```python
from build123d import *

# Parameters (mm, degrees)
SKETCH_1_R      = 1.5
SKETCH_1_R_2    = 1.45
EXTRUDE_1_DEPTH = 4


with BuildPart() as part:
    # 草圖1 → 填料-伸長1 (new body)
    with BuildSketch(Plane(origin=(0, 4, 0), x_dir=(1, 0, 0), z_dir=(0, 1, 0))):
        Polygon((-75, 160.5), (-90, 190.5), (-110, 190.5), (-110, -190.5), (110, -190.5), (110, 190.5), (90, 190.5), (75, 160.5), align=None)
        with Locations((79.5, -32.625)):
            Circle(SKETCH_1_R, mode=Mode.SUBTRACT)
        with Locations((79.5, -140.625)):
            Circle(SKETCH_1_R, mode=Mode.SUBTRACT)
        with Locations((-75, 132.5)):
            Circle(SKETCH_1_R_2, mode=Mode.SUBTRACT)
        with Locations((1.6, 132.5)):
            Circle(SKETCH_1_R_2, mode=Mode.SUBTRACT)
        with Locations((-75, 70.78)):
            Circle(SKETCH_1_R_2, mode=Mode.SUBTRACT)
        with Locations((1.6, 70.78)):
            Circle(SKETCH_1_R_2, mode=Mode.SUBTRACT)
        with Locations((1.6, 55.5)):
            Circle(SKETCH_1_R_2, mode=Mode.SUBTRACT)
        with Locations((-75, 55.5)):
            Circle(SKETCH_1_R_2, mode=Mode.SUBTRACT)
        with Locations((-75, -6.22)):
            Circle(SKETCH_1_R_2, mode=Mode.SUBTRACT)
        with Locations((1.6, -6.22)):
            Circle(SKETCH_1_R_2, mode=Mode.SUBTRACT)
        with Locations((-75, -21.5)):
            Circle(SKETCH_1_R_2, mode=Mode.SUBTRACT)
        with Locations((1.6, -21.5)):
            Circle(SKETCH_1_R_2, mode=Mode.SUBTRACT)
        with Locations((-75, -83.22)):
            Circle(SKETCH_1_R_2, mode=Mode.SUBTRACT)
        with Locations((1.6, -83.22)):
            Circle(SKETCH_1_R_2, mode=Mode.SUBTRACT)
        with Locations((1.6, -98.5)):
            Circle(SKETCH_1_R_2, mode=Mode.SUBTRACT)
        with Locations((-75, -98.5)):
            Circle(SKETCH_1_R_2, mode=Mode.SUBTRACT)
        with Locations((-75, -160.22)):
            Circle(SKETCH_1_R_2, mode=Mode.SUBTRACT)
        with Locations((1.6, -160.22)):
            Circle(SKETCH_1_R_2, mode=Mode.SUBTRACT)
        with Locations((-28.86, -181.5)):
            Circle(SKETCH_1_R_2, mode=Mode.SUBTRACT)
        with Locations((78.5, -181.5)):
            Circle(SKETCH_1_R_2, mode=Mode.SUBTRACT)
        with BuildLine():
            Line((-104, 1.5), (-102, 1.5))
            ThreePointArc((-102, 1.5), (-100.5, 0), (-102, -1.5))
            Line((-102, -1.5), (-104, -1.5))
            ThreePointArc((-104, -1.5), (-105.5, 0), (-104, 1.5))
        make_face(mode=Mode.SUBTRACT)
        with BuildLine():
            Line((102, -116), (104, -116))
            ThreePointArc((104, -116), (105.5, -117.5), (104, -119))
            Line((104, -119), (102, -119))
            ThreePointArc((102, -119), (100.5, -117.5), (102, -116))
        make_face(mode=Mode.SUBTRACT)
        with BuildLine():
            Line((102, 1.5), (104, 1.5))
            ThreePointArc((104, 1.5), (105.5, 0), (104, -1.5))
            Line((104, -1.5), (102, -1.5))
            ThreePointArc((102, -1.5), (100.5, 0), (102, 1.5))
        make_face(mode=Mode.SUBTRACT)
        with BuildLine():
            Line((102, 119), (104, 119))
            ThreePointArc((104, 119), (105.5, 117.5), (104, 116))
            Line((104, 116), (102, 116))
            ThreePointArc((102, 116), (100.5, 117.5), (102, 119))
        make_face(mode=Mode.SUBTRACT)
        with BuildLine():
            Line((-104, -116), (-102, -116))
            ThreePointArc((-102, -116), (-100.5, -117.5), (-102, -119))
            Line((-102, -119), (-104, -119))
            ThreePointArc((-104, -119), (-105.5, -117.5), (-104, -116))
        make_face(mode=Mode.SUBTRACT)
        with BuildLine():
            Line((-104, 119), (-102, 119))
            ThreePointArc((-102, 119), (-100.5, 117.5), (-102, 116))
            Line((-102, 116), (-104, 116))
            ThreePointArc((-104, 116), (-105.5, 117.5), (-104, 119))
        make_face(mode=Mode.SUBTRACT)
        Polygon((15.6, 132.5), (57.6, 132.5), (62.6, 127.5), (62.6, 75.78), (57.6, 70.78), (15.6, 70.78), align=None, mode=Mode.SUBTRACT)
        Polygon((57.6, 55.5), (62.6, 50.5), (62.6, -1.22), (57.6, -6.22), (15.6, -6.22), (15.6, 55.5), align=None, mode=Mode.SUBTRACT)
        Polygon((57.6, -21.5), (62.6, -26.5), (62.6, -78.22), (57.6, -83.22), (15.6, -83.22), (15.6, -21.5), align=None, mode=Mode.SUBTRACT)
        Polygon((57.6, -98.5), (62.6, -103.5), (62.6, -155.22), (57.6, -160.22), (15.6, -160.22), (15.6, -98.5), align=None, mode=Mode.SUBTRACT)
    extrude(amount=-EXTRUDE_1_DEPTH)


solid = part.part
```
The listing builds one solid part. Answer for the finished solid, in the listing's coordinates (mm). A direction names the side the tool comes from. Round coordinates to 2 decimals unless told otherwise and drop trailing zeros. Write each loop counter-clockwise with the first axis right and the second up, starting at its lowest first coordinate (ties: lowest second). Pieces come first, ordered by that corner, then holes. Notation, with made-up numbers: (50, 66) -> (70, 66) arc R19 ccw to (70, 82) -> close; hole circle Ø2 at (67.5, -29.75). An arc over 180 degrees is marked (long way). Write item = value, one per line.
1) Which of the six approach directions +Z, -Z, +X, -X, +Y, -Y give full straight-line access (tool end or side, diameter ignored) to faces 1 (the flat face through (-82.4, 2, -175.3)), 2 (the flat face through (-2, 4, -3))?
Check values:
face_1 = -Z, +Y, -Y
face_2 = +Z, -Z, +X, -X, +Y
2) Section B-B on x = -83 is taken. Write down the section's boundary in (y, z), plus the area to 3 significant figures.
Check values:
outline = (0, -176.5) -> (4, -176.5) -> (4, 190.5) -> (0, 190.5) -> close
area = 1,470 mm²
3) Section C-C on y = 2.15 is taken. Give the number of separate pieces and of enclosed holes in the cut face, plus the area to 3 significant figures.
Check values:
separate_pieces = 1
enclosed_holes = 30
area = 67,200 mm²
4) Straight lines are drawn through the part: line 1 along Z through (x, y) = (-28.86, 2.55); line 2 along X through (y, z) = (1.95, 64.5); line 3 along Z through (x, y) = (79.5, 2) (3 decimals). For each, find the intervals that lie inside material, in ascending order. Write a range as [from, to].
Check values:
line_1 = [-160.5, 180.05], [182.95, 190.5]
line_2 = [-110, 15.6], [62.6, 110]
line_3 = [-169.5, 31.125], [34.125, 139.125], [142.125, 180.45], [182.55, 190.5]
5) Section A-A on z = -27.5 is taken. Write down the section's boundary in (x, y), plus the area to 3 significant figures.
Check values:
outline = (-110, 0) -> (15.6, 0) -> (15.6, 4) -> (-110, 4) -> close; (62.6, 0) -> (110, 0) -> (110, 4) -> (62.6, 4) -> close
area = 692 mm²
